Build history of the part. All positions in model axes, mm. A direction names the side the tool comes from. Give positions to 0.01 mm unless a question says otherwise; leave off trailing zeros. Loops run counter-clockwise (first coordinate to the right, second up) from the corner with the lowest first, then second, coordinate; pieces in that order, holes last. Notation, with made-up numbers: M 68.5,6.5 L 117.5,6.5 A15 ccw 117.5,11.5 Z; hole C -23.75,16 d11. An arc over 180 degrees is marked long. Put each result on its own line as item: value.
```python
from build123d import *

# Parameters (mm, degrees)
SKETCH1_R           = 1
BOSS_EXTRUDE1_DEPTH = 12.7
SKETCH2_R           = 4
CUT_EXTRUDE1_DEPTH  = 10


with BuildPart() as part:
    # Sketch1 → Boss-Extrude1 (new body)
    with BuildSketch(Plane(origin=(0, 0, 0), x_dir=(1, 0, 0), z_dir=(0, 1, 0))):
        with BuildLine():
            Line((-4.055343897, 0.632583633), (-4.075844459, 0.866906139))
            ThreePointArc((-4.075844459, 0.866906139), (-3.83530083, 1.283539926), (-3.361522369, 1.2))
            Line((-3.361522369, 1.2), (-2.761522369, 0.6))
            ThreePointArc((-2.761522369, 0.6), (-2.304491577, 0.509090923), (-2.04560443, 0.89654292))
            Line((-2.04560443, 0.89654292), (-2.04560443, 3))
            ThreePointArc((-2.04560443, 3), (-2.924284086, 5.121320344), (-5.04560443, 6))
            Line((-5.04560443, 6), (-18, 6))
            Line((-18, 6), (-18, -6))
            ThreePointArc((-18, -6), (-15.656854249, -11.656854249), (-10, -14))
            Line((-10, -14), (8.95439557, -14))
            ThreePointArc((8.95439557, -14), (15.318356601, -11.363961031), (17.95439557, -5))
            Line((17.95439557, -5), (17.95439557, -0.89654292))
            ThreePointArc((17.95439557, -0.89654292), (17.695508423, -0.509090923), (17.238477631, -0.6))
            Line((17.238477631, -0.6), (16.638477631, -1.2))
            ThreePointArc((16.638477631, -1.2), (16.16469917, -1.283539926), (15.924155541, -0.866906139))
            Line((15.924155541, -0.866906139), (15.944656103, -0.632583633))
            ThreePointArc((15.944656103, -0.632583633), (15.365, 0), (15.944656103, 0.632583633))
            Line((15.944656103, 0.632583633), (15.924155541, 0.866906139))
            ThreePointArc((15.924155541, 0.866906139), (16.16469917, 1.283539926), (16.638477631, 1.2))
            Line((16.638477631, 1.2), (17.238477631, 0.6))
            ThreePointArc((17.238477631, 0.6), (17.695508423, 0.509090923), (17.95439557, 0.89654292))
            ThreePointArc((17.95439557, 0.89654292), (14.95439557, 3.89654292), (11.95439557, 0.89654292))
            Line((11.95439557, 0.89654292), (11.95439557, -5))
            ThreePointArc((11.95439557, -5), (11.075715914, -7.121320344), (8.95439557, -8))
            Line((8.95439557, -8), (0.95439557, -8))
            ThreePointArc((0.95439557, -8), (-1.166924773, -7.121320344), (-2.04560443, -5))
            Line((-2.04560443, -5), (-2.04560443, -0.89654292))
            ThreePointArc((-2.04560443, -0.89654292), (-2.304491577, -0.509090923), (-2.761522369, -0.6))
            Line((-2.761522369, -0.6), (-3.361522369, -1.2))
            ThreePointArc((-3.361522369, -1.2), (-3.83530083, -1.283539926), (-4.075844459, -0.866906139))
            Line((-4.075844459, -0.866906139), (-4.055343897, -0.632583633))
            ThreePointArc((-4.055343897, -0.632583633), (-4.635, 0), (-4.055343897, 0.632583633))
        make_face()
        with Locations(Location((-8, 0, 0), (0, 0, 270))):
            Circle(SKETCH1_R, mode=Mode.SUBTRACT)
    extrude(amount=BOSS_EXTRUDE1_DEPTH)

    # Sketch2 → Cut-Extrude1 (cut)
    with BuildSketch(Plane.ZY.offset(18)):
        with Locations((0, 6.35)):
            Circle(SKETCH2_R)
    extrude(amount=-CUT_EXTRUDE1_DEPTH, mode=Mode.SUBTRACT)


solid = part.part
```
Q1. Drop flat-ended pins along their axis: pin 1 Ø1.1 at (y, z) = (7, -2) entering from +X; pin 2 Ø3.5 at (y, z) = (6, 2) entering from -X. Give the stop position or say it passes through.
Here are the results:
pin 1: x = 17.9
pin 2: x = -8
Q2. Probe line 1 (X direction, y = 5, z = 0) (3 decimals); line 2 (Y direction, x = -10.75, z = 0); line 3 (X direction, y = 6, z = 4.25). List the from-to ranges inside material, lowest first. Write a range as from..to.
Here are the results:
line 1: -7..-4.635, 11.954..15.365
line 2: 0..2.35, 10.35..12.7
line 3: -18..-2.05, 11.95..17.95
Q3. Slice it at D-D (x = -13). List the corners of the cut face in (y, z), and give its area (3 significant figures).
Here are the results:
outline: M 0,-6 L 12.7,-6 L 12.7,13.42 L 0,13.42 Z; hole C 6.35,0 d8
area: 196 mm²
Q4. Mould opens along X. For faces 1 (the flat face through (-8, 6, -2)), 2 (the cylindrical face through (-1.143, 6.261, 7.145)), 3 (the flat face through (-4, 0, 6)), 4 (the cylindrical face through (15.25, 6.26, 11.43)) say: pulls with the +X half, pulls with the -X half, needs draft (parallel to the pull), parting line crosses it, or undercut.
Here are the results:
face 1: pulls with the -X half
face 2: undercut
face 3: needs draft
face 4: pulls with the +X half
Q5. Tool access for faces 5 (the cylindrical face through (-15.719, 6.261, 11.594)), 6 (the cylindrical face through (11.099, 6.261, 7.098)), 7 (the flat face through (-8, 6, 2)), 8 (the cylindrical face through (15.365, 6.261, 0.013)): list every direction of +Z, -Z, +X, -X, +Y, -Y with a clear straight run to the whole face (end or side of a thin tool).
Here are the results:
face 5: +Z, -X, +Y, -Y
face 6: -Z, +Y, -Y
face 7: -X
face 8: +Y, -Y
Q6. Slice it at C-C (z = 6.75). List the corners of the cut face in (x, y).
Here are the results:
outline: M -17.96,0 L -1.48,0 L -1.48,12.7 L -17.96,12.7 Z; M 11.39,0 L 17.78,0 L 17.78,12.7 L 11.39,12.7 Z
Q7. Slice it at A-A (z = 0). List the corners of the cut face in (x, y) (3 decimals), and give its area (3 significant figures).
Here are the results:
outline: M -18,0 L -9,0 L -9,2.35 L -18,2.35 Z; M -18,10.35 L -9,10.35 L -9,12.7 L -18,12.7 Z; M -7,0 L -4.635,0 L -4.635,12.7 L -7,12.7 Z; M 11.954,0 L 15.365,0 L 15.365,12.7 L 11.954,12.7 Z
area: 116 mm²
